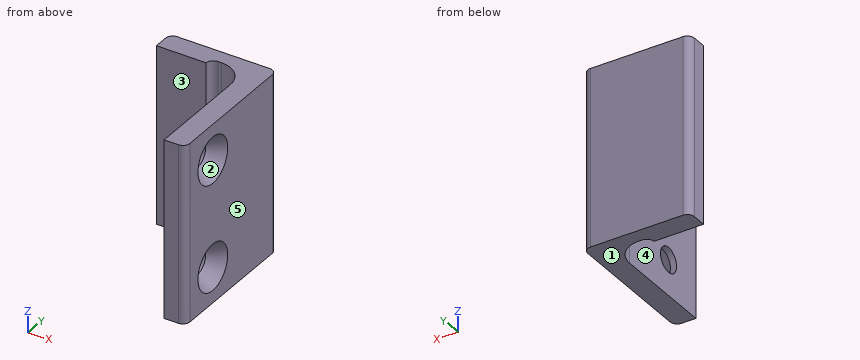
```python
from build123d import *

# Parameters (mm, degrees)
F1_DEPTH       = 25
F3_D           = 3.5
F3_CSINK_D     = 6.5
F3_CSINK_ANGLE = 70


with BuildPart() as f1:
    # F0 (on Top) → F1 (new body)
    with BuildSketch(Plane.XY):
        with BuildLine():
            Line((4.472217, -11.782544), (-8.527783, -11.782544))
            ThreePointArc((-8.527783, -11.782544), (-9.23489, -12.075437), (-9.527783, -12.782544))
            Line((-9.527783, -12.782544), (-9.527783, -14.782544))
            Line((-9.527783, -14.782544), (-2.527783, -14.782544))
            ThreePointArc((-2.527783, -14.782544), (-2.23489, -14.075437), (-1.527783, -13.782544))
            Line((-1.527783, -13.782544), (-1.027783, -13.782544))
            ThreePointArc((-1.027783, -13.782544), (1.447091, -14.80767), (2.472217, -17.282544))
            Line((2.472217, -17.282544), (2.472217, -31.782544))
            Line((2.472217, -31.782544), (4.472217, -31.782544))
            ThreePointArc((4.472217, -31.782544), (5.179324, -31.489651), (5.472217, -30.782544))
            Line((5.472217, -30.782544), (5.472217, -12.782544))
            ThreePointArc((5.472217, -12.782544), (5.179324, -12.075437), (4.472217, -11.782544))
        make_face()
    extrude(amount=F1_DEPTH)

    # F3 (through all)
    with Locations(Plane.YZ.offset(5.472217)):
        with Locations((-25.782544, 20), (-25.782544, 5)):
            CounterSinkHole(F3_D / 2, F3_CSINK_D / 2, counter_sink_angle=F3_CSINK_ANGLE)


solid = f1.part
```
Could you check a few things on this model? Use its own coordinates, in mm. Face numbers are marked on the shaded views. A direction names the side the tool comes from. Coordinates: 2 decimals unless noted, no trailing zeros. Write each loop counter-clockwise with the first axis right and the second up, starting at its lowest first coordinate (ties: lowest second). Pieces come first, ordered by that corner, then holes. Notation, with made-up numbers: (65.25, 26.5) -> (80.25, 26.5) arc R11 ccw to (80.25, 34.5) -> close; hole circle Ø7 at (46, -5). An arc over 180 degrees is marked (long way). Write item = value, one per line. Start each with the question number.
(1) We'd pull the mould along Z, two halves only. Please class the marked faces 1, 2 and 3: released by +Z, released by -Z, zero draft, split by the parting line, or undercut.
(2) Will these pins go through, and if not, where does the flat tip stop? pin 1 (6 mm diameter, centred on y = -22, z = 10, fed in from -X); pin 2 (1 mm diameter, centred on x = -1, z = 9, fed in from -Y); pin 3 (3 mm diameter, centred on y = -28.5, z = 21.5, fed in from +X); pin 4 (5.5 mm diameter, centred on x = -7.5, z = 13.5, fed in from -Y).
(3) Which directions (+Z, -Z, +X, -X, +Y, -Y) give clear straight access to the entire face, cutting with the end or side of a thin tool? Please do the marked faces 4 and 5.
(4) I want a section at A-A (z = 20). Please give me the cut outline in (x, y).
(5) I want a section at D-D (y = -24.75). Give the number of separate pieces and of enclosed holes in the cut face, plus the area to 3 significant figures.
(6) I need wall thicknesses on line 1 (Y direction, x = 3.1, z = 5); line 2 (X direction, y = -30, z = 17); line 3 (Y direction, x = -1.25, z = 8.5). Which ranges of each line are inside material? Lowest first, please. Write a range as [from, to].
(7) I want a section at C-C (z = 10.25). Please give me the cut outline in (x, y).
(8) I want a section at B-B (x = 3). Please give me the cut outline in (y, z), plus the area to 3 significant figures.
Result set:
q1.face_1 = released by -Z
q1.face_2 = undercut
q1.face_3 = zero draft
q2.pin_1 = 2.47
q2.pin_2 = -13.82
q2.pin_3 = 5.47
q2.pin_4 = -14.78
q3.face_4 = +Z, -Z, -X, -Y
q3.face_5 = +Z, -Z, +X, +Y, -Y
q4.outline = (-9.53, -14.78) -> (-2.53, -14.78) arc R1 cw to (-1.53, -13.78) -> (-1.03, -13.78) arc R3.5 cw to (2.47, -17.28) -> (2.47, -24.03) -> (3.33, -24.03) -> (5.47, -22.53) -> (5.47, -12.78) arc R1 ccw to (4.47, -11.78) -> (-8.53, -11.78) arc R1 ccw to (-9.53, -12.78) -> close; (2.47, -31.78) -> (4.47, -31.78) arc R1 ccw to (5.47, -30.78) -> (5.47, -29.03) -> (3.33, -27.53) -> (2.47, -27.53) -> close
q5.separate_pieces = 3
q5.enclosed_holes = 0
q5.area = 50.7 mm2
q6.line_1 = [-31.78, -27.53], [-24.03, -11.78]
q6.line_2 = [2.47, 5.47]
q6.line_3 = [-13.78, -11.78]
q7.outline = (-9.53, -14.78) -> (-2.53, -14.78) arc R1 cw to (-1.53, -13.78) -> (-1.03, -13.78) arc R3.5 cw to (2.47, -17.28) -> (2.47, -31.78) -> (4.47, -31.78) arc R1 ccw to (5.47, -30.78) -> (5.47, -12.78) arc R1 ccw to (4.47, -11.78) -> (-8.53, -11.78) arc R1 ccw to (-9.53, -12.78) -> close
q8.outline = (-31.78, 0) -> (-11.78, 0) -> (-11.78, 25) -> (-31.78, 25) -> close; hole circle Ø3.5 at (-25.78, 5); hole circle Ø3.5 at (-25.78, 20)
q8.area = 481 mm2
